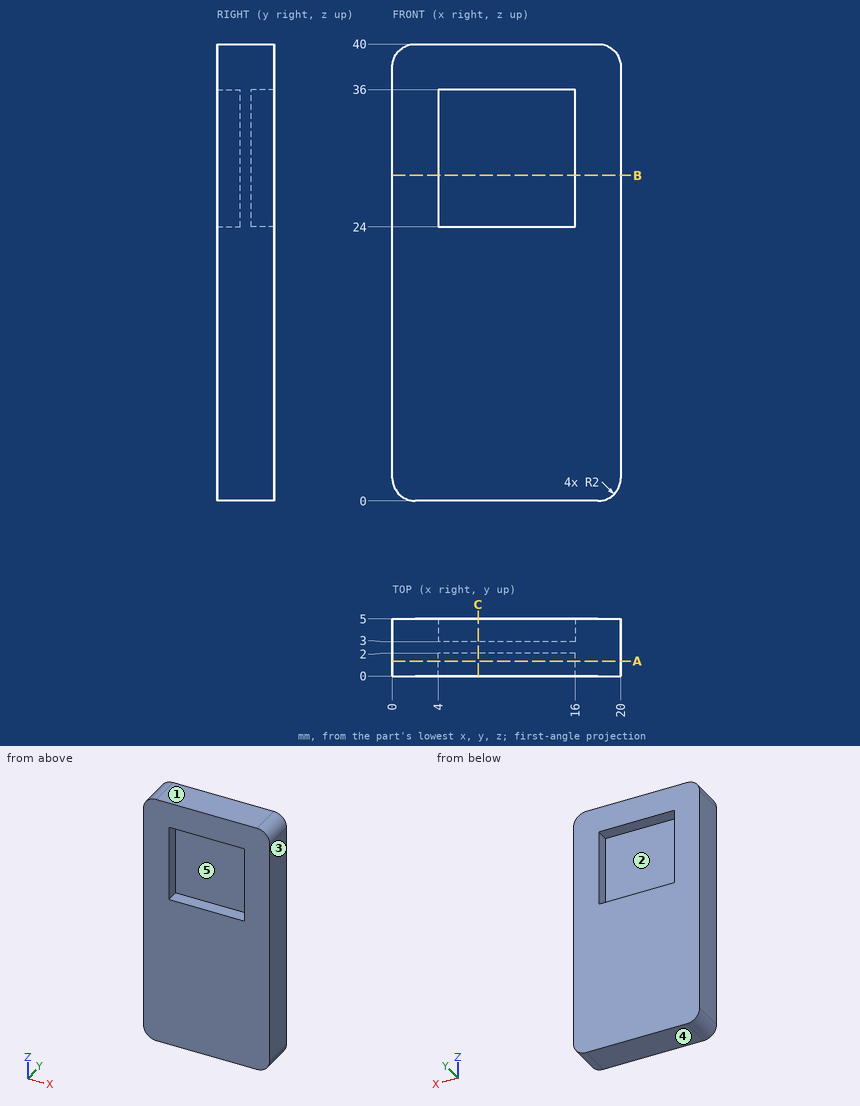
Source: three-view drawing plus pictorial views. Frame: mm from the lowest corner of the part. A direction names the side the tool comes from. Give positions to 0.01 mm unless a question says otherwise; leave off trailing zeros. Write each loop counter-clockwise with the first axis right and the second up, starting at its lowest first coordinate (ties: lowest second). Pieces come first, ordered by that corner, then holes.
(1) Cut plane A-A, the plane y = 1.3. Return loops of the section in (x, z), then the cut area to 3 significant figures.
(2) Cut plane B-B, the plane z = 28.5. Return loops of the section in (x, y).
(3) Cut plane C-C, the plane x = 7.5. Return loops of the section in (y, z).
(4) First-contact query: P1, Ø8, axis at x = 11.5, z = 33.5, coming from the -Y side; P2, Ø2, axis at x = 9.5, z = 30, coming from the +Y side. Flat tips, straight axial feed; report the tip coordinate or a pass-through.
(5) Ray query, line 1 (Z direction, x = 5.25, y = 1.1); line 2 (Y direction, x = 13.5, z = 35); line 3 (Z direction, x = 18.75, y = 2.45). Return the intervals inside material, ascending.
(6) Mould query, pull axis X, two halves, no side actions, for the marked faces 3, 4 and 5. Classes: released by +X, released by -X, zero draft, split by the parting line, or undercut.
(7) Access query for the marked faces 1 and 2. Directions: +Z, -Z, +X, -X, +Y, -Y. A direction counts if a zero-diameter tool reaches every point of the face in a straight line with its end or side. Return the directions, or none.
Values follow:
1. outline: (0, 2) arc R2 ccw to (2, 0) - (18, 0) arc R2 ccw to (20, 2) - (20, 38) arc R2 ccw to (18, 40) - (2, 40) arc R2 ccw to (0, 38) - close; hole (4, 24) - (16, 24) - (16, 36) - (4, 36) - close
1. area: 653 mm2
2. outline: (0, 0) - (4, 0) - (4, 2) - (16, 2) - (16, 0) - (20, 0) - (20, 5) - (16, 5) - (16, 3) - (4, 3) - (4, 5) - (0, 5) - close
3. outline: (0, 0) - (5, 0) - (5, 24) - (3, 24) - (3, 36) - (5, 36) - (5, 40) - (0, 40) - (0, 36) - (2, 36) - (2, 24) - (0, 24) - close
4. P1: stops at y = 0
4. P2: stops at y = 3
5. line 1: z = 0 to 24, 36 to 40
5. line 2: y = 2 to 3
5. line 3: z = 0.15 to 39.85
6. face 3: released by +X
6. face 4: zero draft
6. face 5: undercut
7. face 1: +Z, +X, -X, +Y, -Y
7. face 2: +Y
